Verification items for the finished model (mm, model axes). A direction names the side the tool comes from. Coordinates: 2 decimals unless noted, no trailing zeros. Write each loop counter-clockwise with the first axis right and the second up, starting at its lowest first coordinate (ties: lowest second). Pieces come first, ordered by that corner, then holes. Notation, with made-up numbers: M 68,-11 L 74,-11 A18 ccw 74,13 Z; hole C -15.5,83 d9. An arc over 180 degrees is marked long. Answer in a Markdown table with one row per item.
from build123d import *

# Parameters (mm, degrees)
BOSS_EXTRUDE1_DEPTH = 18.3134
SKETCH2_R           = 3.9624
CUT_EXTRUDE1_DEPTH  = 10.271
SKETCH3_R           = 3.81
CUT_EXTRUDE2_DEPTH  = 6.35


with BuildPart() as part:
    # Sketch1 → Boss-Extrude1 (new body)
    with BuildSketch(Plane.XY):
        Polygon((0, 0), (0, 14.351), (8.0518, 14.351), (13.3858, 9.271), (27.1145, 9.271), (27.1145, 0), align=None)
    extrude(amount=BOSS_EXTRUDE1_DEPTH)

    # Sketch2 → Cut-Extrude1 (cut, through all)
    with BuildSketch(Plane(origin=(0, 9.271, 0), x_dir=(1, 0, 0), z_dir=(0, 1, 0))):
        with Locations(Location((18.0721, -9.1567, 0), (0, 0, 180))):  # turned: the seam where the file's is
            Circle(SKETCH2_R)
    extrude(amount=-CUT_EXTRUDE1_DEPTH, mode=Mode.SUBTRACT)

    # Sketch3 → Cut-Extrude2 (cut)
    with BuildSketch(Plane.ZY):
        with Locations((9.1567, 6.096)):
            Circle(SKETCH3_R)
    extrude(amount=-CUT_EXTRUDE2_DEPTH, mode=Mode.SUBTRACT)


solid = part.part
1) Tool access check on faces 5 (the face through (6.35, 6, 9)), 6 (the face through (22, 9.271, 7)), 7 (the face through (0, 10.3, 9)). Record the directions out of +Z, -Z, +X, -X, +Y, -Y that give a thin tool (end or side, any length) a straight path to the whole face; none if there is none.
Response values:
| item | result |
|---|---|
| face 5 | -X |
| face 6 | +Z, -Z, +X, +Y |
| face 7 | +Z, -Z, -X, +Y, -Y |
2) Sectioned sample at D-D (x = 17.75). Record the cut outline in (y, z), then the cut area to 3 significant figures.
Response values:
| item | result |
|---|---|
| outline | M 0,0 L 9.27,0 L 9.27,5.21 L 0,5.21 Z; M 0,13.11 L 9.27,13.11 L 9.27,18.31 L 0,18.31 Z |
| area | 96.6 mm² |
3) Sectioned sample at A-A (z = 11.5). Record the cut outline in (x, y), then the cut area to 3 significant figures.
Response values:
| item | result |
|---|---|
| outline | M 0,0 L 14.88,0 L 14.88,9.27 L 13.39,9.27 L 8.05,14.35 L 0,14.35 L 0,9.1 L 6.35,9.1 L 6.35,3.09 L 0,3.09 Z; M 21.27,0 L 27.11,0 L 27.11,9.27 L 21.27,9.27 Z |
| area | 208 mm² |
4) Sectioned sample at B-B (y = 3.5). Record the cut outline in (x, z).
Response values:
| item | result |
|---|---|
| outline | M 0,0 L 27.11,0 L 27.11,18.31 L 0,18.31 L 0,11.95 L 6.35,11.95 L 6.35,6.37 L 0,6.37 Z; hole C 18.07,9.16 d7.92 |
5) Sectioned sample at C-C (z = 15). Record the cut outline in (x, y), then the cut area to 3 significant figures.
Response values:
| item | result |
|---|---|
| outline | M 0,0 L 27.11,0 L 27.11,9.27 L 13.39,9.27 L 8.05,14.35 L 0,14.35 Z |
| area | 306 mm² |
6) Depth check by flat-ended pin: pin 1 (8.5 mm diameter, centred on y = 6.5, z = 9.5, fed in from -X); pin 2 (9 mm diameter, centred on x = 18.07, z = 9.16, fed in from +Y). Enter the tip coordinate at first touch or a pass-through.
Response values:
| item | result |
|---|---|
| pin 1 | stops at x = 0 |
| pin 2 | stops at y = 9.27 |
7) Thickness scan on L1, parallel to X at y = 9, z = 9.25; L2, parallel to Y at x = 24.5, z = 15.5; L3, parallel to Z at x = 3.5, y = 5. Record the ranges inside material, lowest first. Write a range as [from, to].
Response values:
| item | result |
|---|---|
| L1 | x = [6.35, 14.11], [22.03, 27.11] |
| L2 | y = [0, 9.27] |
| L3 | z = [0, 5.51], [12.81, 18.31] |
8) Release check for a two-part mould opening along Z. For faces 1 (the face through (14, 6, 0)), 2 (the face through (18.93, 4.7, 5.29)), 3 (the face through (14, 6, 18.313)), 4 (the face through (3.13, 7.24, 12.79)) record: +Z half, -Z half, draft (parallel to the pull), parting line (faces both ways), or undercut.
Response values:
| item | result |
|---|---|
| face 1 | -Z half |
| face 2 | undercut |
| face 3 | +Z half |
| face 4 | undercut |
